Design review of the part built by this model. Coordinates are the model's own, in mm. Coordinates: 2 decimals unless noted, no trailing zeros. Loops run counter-clockwise (first coordinate to the right, second up) from the corner with the lowest first, then second, coordinate; pieces in that order, holes last. Notation, with made-up numbers: M 25,69.25 L 54,69.25 A18 cw 54,100.25 Z; hole C 25,47 d11. An arc over 180 degrees is marked long. Put each result on its own line as item: value. Start each with the question number.
(1) Take a section at A-A, the plane y = 0. Give the boundary of the cut face in (x, z), then the cut area to 3 significant figures.
(2) The part is to be moulded in two halves that separate along X. For faces 1 (the flat face through (13, 0, 0)), 2 (the cylindrical face through (-4.76, 0.1, 1.25)), 3 (the cylindrical face through (24.564, 0.112, 1.252)), say which applies: +X half, -X half, draft (parallel to the pull), parting line (faces both ways), or undercut.
(3) For probe 1 along X at (y, z) = (0.5, 2.2); probe 2 along X at (y, z) = (-0.75, 1.45); probe 3 along Y at (x, z) = (25.5, 1.6), list the stretches that pass through material, from the lowest coordinate up. Write a range as [from, to].
(4) Take a section at B-B, the plane z = 0.6. Give the boundary of the cut face in (x, y) (1 decimal).
(5) Take a section at D-D, the plane y = 3. Give the boundary of the cut face in (x, z).
(6) Take a section at C-C, the plane y = -2. Give the boundary of the cut face in (x, z).
```python
from build123d import *

# Parameters (mm, degrees)
SKETCH1_R           = 4.7625
SKETCH1_R_2         = 1.5875
SKETCH1_R_3         = 2.54
BOSS_EXTRUDE2_DEPTH = 2.54


with BuildPart() as part:
    # Sketch1 → Boss-Extrude2 (new body)
    # profile 1 of 3: a face of its own
    with BuildSketch(Plane.XY):
        Circle(SKETCH1_R)
        Circle(SKETCH1_R_2, mode=Mode.SUBTRACT)
    # profile 2 of 3: a face of its own
    with BuildSketch(Plane.XY):
        with Locations((27.1018, 0)):
            Circle(SKETCH1_R)
        with Locations((27.1018, 0)):
            Circle(SKETCH1_R_3, mode=Mode.SUBTRACT)
    # profile 3 of 3: a face of its own
    with BuildSketch(Plane.XY):
        with BuildLine():
            Line((27.1018, 4.7625), (0, 4.7625))
            ThreePointArc((0, 4.7625), (3.367596045, 3.367596045), (4.7625, 0))
            ThreePointArc((4.7625, 0), (3.367596045, -3.367596045), (0, -4.7625))
            Line((0, -4.7625), (27.1018, -4.7625))
            ThreePointArc((27.1018, -4.7625), (22.3393, 0), (27.1018, 4.7625))
        make_face()
    extrude(amount=BOSS_EXTRUDE2_DEPTH)


solid = part.part
```
Computed values:
1. outline: M -4.76,0 L -1.59,0 L -1.59,2.54 L -4.76,2.54 Z; M 1.59,0 L 24.56,0 L 24.56,2.54 L 1.59,2.54 Z; M 29.64,0 L 31.86,0 L 31.86,2.54 L 29.64,2.54 Z
1. area: 72.1 mm^2
2. face 1: draft
2. face 2: -X half
2. face 3: undercut
3. probe 1: x = [-4.74, -1.51], [1.51, 24.61], [29.59, 31.84]
3. probe 2: x = [-4.7, -1.4], [1.4, 24.68], [29.53, 31.8]
3. probe 3: y = [-4.76, -1.97], [1.97, 4.76]
4. outline: M 0,-4.8 L 27.1,-4.8 A4.8 ccw 27.1,4.8 L 0,4.8 A4.8 ccw Z; hole C 0,0 d3.2; hole C 27.1,0 d5.1
5. outline: M -3.7,0 L 30.8,0 L 30.8,2.54 L -3.7,2.54 Z
6. outline: M -4.32,0 L 25.54,0 L 25.54,2.54 L -4.32,2.54 Z; M 28.67,0 L 31.42,0 L 31.42,2.54 L 28.67,2.54 Z
